Could you check a few things on this model? Use its own coordinates, in mm. Face numbers are marked on the shaded views. A direction names the side the tool comes from. Round coordinates to 2 decimals unless told otherwise and drop trailing zeros. Loops run counter-clockwise (first coordinate to the right, second up) from the corner with the lowest first, then second, coordinate; pieces in that order, holes last. Notation, with made-up numbers: (50, 35) - (83, 35) arc R25 cw to (83, 73) - close; hole circle Ø10 at (50.5, 66.5). An arc over 180 degrees is marked (long way). Use one line per item in the form item = value.
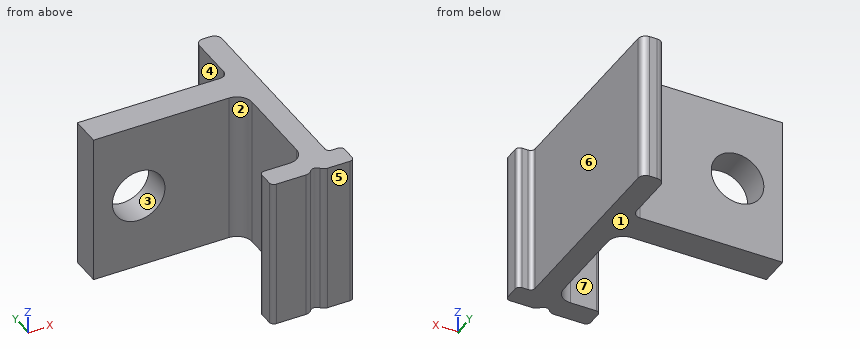
```python
from build123d import *

# Parameters (mm, degrees)
BOSS_EXTRUDE1_DEPTH  = 10
FILLET1_R            = 0.5
M3_CLEARANCE_HOLE1_D = 3.5
CUT_EXTRUDE1_DEPTH   = 10


with BuildPart() as part:
    # Sketch1 → Boss-Extrude1 (new body)
    with BuildSketch(Plane.XY):
        with BuildLine():
            Line((0, 0), (9.5, 0))
            ThreePointArc((9.5, 0), (9.853553391, 0.146446609), (10, 0.5))
            Line((10, 0.5), (10, 3.5))
            ThreePointArc((10, 3.5), (10.146446609, 3.853553391), (10.5, 4))
            Line((10.5, 4), (11, 4))
            ThreePointArc((11, 4), (11.353553391, 3.853553391), (11.5, 3.5))
            Line((11.5, 3.5), (11.5, -9.2))
            ThreePointArc((11.5, -9.2), (11.587867966, -9.412132034), (11.8, -9.5))
            Line((11.8, -9.5), (12.2, -9.5))
            ThreePointArc((12.2, -9.5), (12.412132034, -9.587867966), (12.5, -9.8))
            Line((12.5, -9.8), (12.5, -10.7))
            ThreePointArc((12.5, -10.7), (12.412132034, -10.912132034), (12.2, -11))
            Line((12.2, -11), (10.375, -11))
            ThreePointArc((10.375, -11), (10, -10.625), (9.625, -11))
            Line((9.625, -11), (7.3, -11))
            ThreePointArc((7.3, -11), (7.087867966, -10.912132034), (7, -10.7))
            Line((7, -10.7), (7, -9.8))
            ThreePointArc((7, -9.8), (7.070871215, -9.606350833), (7.25, -9.504196011))
            ThreePointArc((7.25, -9.504196011), (7.429128785, -9.402041189), (7.5, -9.208392022))
            Line((7.5, -9.208392022), (7.5, -2.2))
            ThreePointArc((7.5, -2.2), (7.441421356, -2.058578644), (7.3, -2))
            Line((7.3, -2), (0, -2))
            Line((0, -2), (0, 0))
        make_face()
    extrude(amount=BOSS_EXTRUDE1_DEPTH)

    # Fillet1
    fillet1_edges = [part.edges().sort_by_distance(p)[0] for p in [
        (10.375, -11, 5),
        (9.625, -11, 5),
    ]]
    fillet(fillet1_edges, radius=FILLET1_R)

    # M3 Clearance Hole1 (through all)
    with Locations(Plane(origin=(0, 0, 0), x_dir=(1, 0, 0), z_dir=(0, 1, 0))):
        with Locations((3, -5)):
            Hole(M3_CLEARANCE_HOLE1_D / 2)

    # Sketch4 → Cut-Extrude1 (cut)
    with BuildSketch(Plane.XY.offset(10)):
        with BuildLine():
            Line((7.25, -9.504196011), (9, -9.504196011))
            ThreePointArc((9, -9.504196011), (9.707106781, -9.211302792), (10, -8.504196011))
            Line((10, -8.504196011), (10, -3))
            ThreePointArc((10, -3), (9.707106781, -2.292893219), (9, -2))
            Line((9, -2), (7.5, -2))
            Line((7.5, -2), (7.25, -2))
            Line((7.25, -2), (7.25, -9.504196011))
        make_face()
    extrude(amount=-CUT_EXTRUDE1_DEPTH, mode=Mode.SUBTRACT)


solid = part.part
```
1. If we section it at D-D, the plane y = -8.25: Write out the boundary of the cut face in (x, z), plus the area to 3 significant figures.
Solution:
outline = (10, 0) - (11.5, 0) - (11.5, 10) - (10, 10) - close
area = 15.0 mm^2
2. If we section it at C-C, the plane x = 3: Write out the boundary of the cut face in (y, z), plus the area to 3 significant figures.
Solution:
outline = (-2, 0) - (0, 0) - (0, 3.25) - (-2, 3.25) - close; (-2, 6.75) - (0, 6.75) - (0, 10) - (-2, 10) - close
area = 13.0 mm^2
3. For P1, Ø0.9, axis at y = 1.5, z = 6.5, coming from the -X side; P2, Ø5, axis at x = 2.5, z = 7, coming from the -Y side; P3, Ø3, axis at x = 6, z = 8, coming from the -Y side; P4, Ø1, axis at x = 7.5, z = 7, coming from the +Y side, each with a flat end and sliding along its axis, tell me the tip position at first contact or that it passes through.
Solution:
P1 = 10
P2 = -2
P3 = -11
P4 = 0
4. On a 3-axis mill with a long thin cutter (end or side, diameter ignored), from which of +Z, -Z, +X, -X, +Y, -Y can I reach the whole of each face in a straight line? I mean the marked faces 4, 5, 6 and 7. Say none if no direction works.
Solution:
face_4 = +Z, -Z, -X, +Y
face_5 = +Z, -Z, +X, -X, -Y
face_6 = +Z, -Z, +X, +Y
face_7 = +Z, -Z, -X
5. We'd pull the mould along Z, two halves only. Please class the marked faces 1, 2 and 3: +Z half, -Z half, draft (parallel to the pull), parting line (faces both ways), or undercut.
Solution:
face_1 = -Z half
face_2 = draft
face_3 = undercut
6. If we section it at A-A, the plane x = 8.5: Write out the boundary of the cut face in (y, z), plus the area to 3 significant figures.
Solution:
outline = (-11, 0) - (-9.5, 0) - (-9.5, 10) - (-11, 10) - close; (-2, 0) - (0, 0) - (0, 10) - (-2, 10) - close
area = 35.0 mm^2
7. Please list where these lines run through material, in increasing order: line 1 along Z through (x, y) = (3, -0.8); line 2 along Y through (x, z) = (9, 0.75); line 3 along X through (y, z) = (-0.6, 5).
Solution:
line_1 = 0 to 3.25, 6.75 to 10
line_2 = -11 to -9.5, -2 to 0
line_3 = 0 to 1.25, 4.75 to 11.5
